from build123d import *

# Parameters (mm, degrees)
SKETCH1_R           = 60
BOSS_EXTRUDE1_DEPTH = 50
FILLET1_R           = 5
SKETCH2_R           = 35.344502653
CUT_EXTRUDE1_DEPTH  = 5
SKETCH3_R           = 2.5
CUT_EXTRUDE2_DEPTH  = 97.046863624


with BuildPart() as part:
    # Sketch1 → Boss-Extrude1 (new body)
    with BuildSketch(Plane.XY):
        Circle(SKETCH1_R)
    extrude(amount=BOSS_EXTRUDE1_DEPTH)

    # Fillet1
    fillet1_edges = [part.edges().sort_by_distance(p)[0] for p in [
        (-60, 0, 0),
        (-60, 0, 50),
    ]]
    fillet(fillet1_edges, radius=FILLET1_R)

    # Sketch2 → Cut-Extrude1 (cut)
    with BuildSketch(Plane.XY.offset(50)):
        Circle(SKETCH2_R)
    extrude(amount=-CUT_EXTRUDE1_DEPTH, mode=Mode.SUBTRACT)

    # Sketch3 → Cut-Extrude2 (cut, through all)
    with BuildSketch(Plane.XY.offset(45)):
        Circle(SKETCH3_R)
    extrude(amount=-CUT_EXTRUDE2_DEPTH, mode=Mode.SUBTRACT)


solid = part.part
Check sheet for the modelled part. Datum: model origin and axes. Units: mm. A direction names the side the tool comes from. Give positions to 0.01 mm unless a question says otherwise; leave off trailing zeros. Write each loop counter-clockwise with the first axis right and the second up, starting at its lowest first coordinate (ties: lowest second). Pieces come first, ordered by that corner, then holes. Notation, with made-up numbers: (46, 89) -> (67, 89) arc R34 ccw to (67, 120) -> close; hole circle Ø2 at (-39.75, 60). An arc over 180 degrees is marked (long way). Use one line per item in the form item = value. Start each with the question number.
1. Section check A-A (y = 0). Record the cut outline in (x, z), and give its area (3 significant figures).
2. Mould release check, pull along X, two halves, no side actions. Record for faces 1 (the flat face through (-1, -36, 50)), 2 (the cylindrical face through (-59.94, 2.64, 24.72)), 3 (the flat face through (0, -7, 45)): pulls with the +X half, pulls with the -X half, needs draft (parallel to the pull), parting line crosses it, or undercut.
3. Thickness scan on line 1 along Y through (x, z) = (0, 46); line 2 along Z through (x, y) = (38, -40); line 3 along Z through (x, y) = (-25.5, -20). Record the ranges inside material, lowest first. Write a range as from..to.
4. Section check C-C (z = 36.5). Record the cut outline in (x, y), and give its area (3 significant figures).
5. Access from +Z, -Z, +X, -X, +Y, -Y to the whole of each face (thin tool, end or side, straight path). Record for faces 4 (the cylindrical face through (-7.662, -34.504, 47.535)), 5 (the cylindrical face through (-0.54, -2.44, 22.82)).
6. Go/stop test with flat-tipped pins: P1, Ø3, axis at x = -26, z = 44.5, coming from the +Y side; P2, Ø21, axis at x = 7, y = 15, coming from the +Z side; P3, Ø1.5, axis at y = 32.5, z = 23.5, coming from the -X side. Record where each tip stops, or that it passes through.
Conclusion:
q1.outline = (-60, 5) arc R5 ccw to (-55, 0) -> (-2.5, 0) -> (-2.5, 45) -> (-35.34, 45) -> (-35.34, 50) -> (-55, 50) arc R5 ccw to (-60, 45) -> close; (2.5, 0) -> (55, 0) arc R5 ccw to (60, 5) -> (60, 45) arc R5 ccw to (55, 50) -> (35.34, 50) -> (35.34, 45) -> (2.5, 45) -> close
q1.area = 5,400 mm²
q2.face_1 = needs draft
q2.face_2 = parting line crosses it
q2.face_3 = undercut
q3.line_1 = -59.9..-35.34, 35.34..59.9
q3.line_2 = 0..50
q3.line_3 = 0..45
q4.outline = circle Ø120 at (0, 0); hole circle Ø5 at (0, 0)
q4.area = 11,300 mm²
q5.face_4 = +Z
q5.face_5 = +Z, -Z
q6.P1 = 54.77
q6.P2 = 45
q6.P3 = -50.91
